```python
from build123d import *

# Parameters (mm, degrees)
HOLE_D             = 6.6
HOLE_CBORE_D       = 11
HOLE_CBORE_DEPTH   = 6.4
POLARPATTERN_COUNT = 4


with BuildPart() as part:
    # Sketch → Revolution (revolve)
    with BuildSketch(Plane.YZ):
        Polygon((6, 100), (12, 100), (12, 88), (15, 88), (15, 85), (8, 85), (8, 28.5), (23, 28.5), (23, 23.5), (10, 23.5), (10, 21.5), (7, 21.5), (7, 12.5), (0, 12.5), (0, 27.5), (2, 27.5), (2, 67.5), (4, 67.5), (4, 98), align=None)
    revolve(axis=Axis((0, 0, 0), (0, 1, 0)))

    # Hole (through all)
    with Locations(Plane.XZ):
        with Locations((0, 93.5)):
            hole = CounterBoreHole(HOLE_D / 2, HOLE_CBORE_D / 2, HOLE_CBORE_DEPTH)

    # PolarPattern: Hole ×4 about axis
    polarpattern_axis = Axis((0, 0, 0), (0, 1, 0))
    for i in range(1, POLARPATTERN_COUNT):
        add(hole.rotate(polarpattern_axis, i * 360 / POLARPATTERN_COUNT), mode=Mode.SUBTRACT)


solid = part.part
```
Model file for the job. Use its own axes, mm. A direction names the side the tool comes from. Coordinates: 2 decimals unless noted, no trailing zeros. Use CSV: the item, a comma, the result in double quotes. Start each with the question number.
1. Probe probe 1 along X at (y, z) = (12.25, 0); probe 2 along X at (y, z) = (8.65, 0); probe 3 along X at (y, z) = (14, -69.5). List the from-to ranges inside material, lowest first. Write a range as [from, to].
2. Tool access for faces 1 (the cylindrical face through (-96.283, 9.239, -1.774)), 2 (the cylindrical face through (-41.07, 3.01, -53.57)), 3 (the cylindrical face through (-85.907, 13.521, -19.077)): list every direction of +Z, -Z, +X, -X, +Y, -Y with a clear straight run to the whole face (end or side of a thin tool).
3. Band-saw the part on A-A, the plane z = 0. Give the number of separate pieces and of enclosed holes in the cut face, then the cut area to 3 significant figures.
4. Flat gauge pins, fed straight in: pin 1 (1.5 mm diameter, centred on x = -79, y = 14.5, fed in from +Z); pin 2 (9 mm diameter, centred on x = 93.5, z = 1.5, fed in from -Y); pin 3 (4 mm diameter, centred on x = 69.5, y = 16, fed in from +Z). Where does each tip first touch, or does it go through?
Entries:
1,probe 1,"x = [-88, -85], [-28.5, -23.5], [23.5, 28.5], [85, 88]"
1,probe 2,"x = [-100, -96.8], [-90.2, -85], [-28.5, -21.5], [21.5, 28.5], [85, 90.2], [96.8, 100]"
1,probe 3,"x = [-53.98, -48.94], [48.94, 53.98]"
2,face 1,"+Y, -Y"
2,face 2,"-Y"
2,face 3,"+Y"
3,separate pieces,"4"
3,enclosed holes,"0"
3,area,"1,130 mm2"
4,pin 1,"stops at z = 40.26"
4,pin 2,"stops at y = 4"
4,pin 3,"stops at z = 56.14"
